from build123d import *

# Parameters (mm, degrees)
SKETCH1_W           = 40
SKETCH1_H           = 40
BOSS_EXTRUDE1_DEPTH = 60
SKETCH2_W           = 20
SKETCH2_H           = 40
CUT_EXTRUDE1_DEPTH  = 30
SKETCH4_W           = 40
SKETCH4_H           = 30
CUT_EXTRUDE2_DEPTH  = 20
SKETCH5_W           = 30
SKETCH5_H           = 10
CUT_EXTRUDE3_DEPTH  = 15
SKETCH6_W           = 15
SKETCH6_H           = 10
CUT_EXTRUDE4_DEPTH  = 25
SKETCH8_W           = 30
SKETCH8_H           = 15
BOSS_EXTRUDE2_DEPTH = 10
SKETCH10_W          = 30
SKETCH10_H          = 25
CUT_EXTRUDE5_DEPTH  = 5
SKETCH11_W          = 30
SKETCH11_H          = 15
CUT_EXTRUDE6_DEPTH  = 5


with BuildPart() as part:
    # Sketch1 → Boss-Extrude1 (new body)
    with BuildSketch(Plane.XY):
        with Locations((20, 20)):
            Rectangle(SKETCH1_W, SKETCH1_H)
    extrude(amount=BOSS_EXTRUDE1_DEPTH)

    # Sketch2 → Cut-Extrude1 (cut)
    with BuildSketch(Plane.XY.offset(60)):
        with Locations((30, 20)):
            Rectangle(SKETCH2_W, SKETCH2_H)
    extrude(amount=-CUT_EXTRUDE1_DEPTH, mode=Mode.SUBTRACT)

    # Sketch4 → Cut-Extrude2 (cut)
    with BuildSketch(Plane(origin=(0, 40, 0), x_dir=(1, 0, 0), z_dir=(0, 1, 0))):
        with Locations((20, -15)):
            Rectangle(SKETCH4_W, SKETCH4_H)
    extrude(amount=-CUT_EXTRUDE2_DEPTH, mode=Mode.SUBTRACT)

    # Sketch5 → Cut-Extrude3 (cut)
    with BuildSketch(Plane(origin=(40, 0, 0), x_dir=(0, 0, -1), z_dir=(1, 0, 0))):
        with Locations((-15, 5)):
            Rectangle(SKETCH5_W, SKETCH5_H)
    extrude(amount=-CUT_EXTRUDE3_DEPTH, mode=Mode.SUBTRACT)

    # Sketch6 → Cut-Extrude4 (cut)
    with BuildSketch(Plane(origin=(20, 0, 0), x_dir=(0, 0, -1), z_dir=(1, 0, 0))):
        with Locations((-52.5, 35)):
            Rectangle(SKETCH6_W, SKETCH6_H)
    extrude(amount=-CUT_EXTRUDE4_DEPTH, mode=Mode.SUBTRACT)

    # Sketch8 → Boss-Extrude2 (add)
    with BuildSketch(Plane(origin=(20, 0, 0), x_dir=(0, 0, -1), z_dir=(1, 0, 0))):
        with Locations((-45, 7.5)):
            Rectangle(SKETCH8_W, SKETCH8_H)
    extrude(amount=BOSS_EXTRUDE2_DEPTH)

    # Sketch10 → Cut-Extrude5 (cut)
    with BuildSketch(Plane(origin=(20, 0, 0), x_dir=(0, 0, -1), z_dir=(1, 0, 0))):
        with Locations((-45, 27.5)):
            Rectangle(SKETCH10_W, SKETCH10_H)
    extrude(amount=-CUT_EXTRUDE5_DEPTH, mode=Mode.SUBTRACT)

    # Sketch11 → Cut-Extrude6 (cut)
    with BuildSketch(Plane(origin=(30, 0, 0), x_dir=(0, 0, -1), z_dir=(1, 0, 0))):
        with Locations((-45, 7.5)):
            Rectangle(SKETCH11_W, SKETCH11_H)
    extrude(amount=-CUT_EXTRUDE6_DEPTH, mode=Mode.SUBTRACT)


solid = part.part
Verification items for the finished model (mm, model axes). A direction names the side the tool comes from. Round coordinates to 2 decimals unless told otherwise and drop trailing zeros. Loops run counter-clockwise (first coordinate to the right, second up) from the corner with the lowest first, then second, coordinate; pieces in that order, holes last. Notation, with made-up numbers: (-4.5, 32) - (46.5, 32) arc R19 ccw to (46.5, 41) - close; hole circle Ø11 at (14, 80). An arc over 180 degrees is marked (long way). Write item = value, one per line.
Q1. Sectioned sample at C-C on y = 16. Record the boundary of the cut face in (x, z), plus the area to 3 significant figures.
Here are the results:
outline = (0, 0) - (40, 0) - (40, 30) - (15, 30) - (15, 60) - (0, 60) - close
area = 1,650 mm^2
Q2. Sectioned sample at A-A on x = 4. Record the boundary of the cut face in (y, z), plus the area to 3 significant figures.
Here are the results:
outline = (0, 0) - (20, 0) - (20, 30) - (40, 30) - (40, 45) - (30, 45) - (30, 60) - (0, 60) - close
area = 1,650 mm^2
Q3. Depth check by flat-ended pin: pin 1 (8 mm diameter, centred on x = 33.5, z = 12, fed in from +Y); pin 2 (4.5 mm diameter, centred on x = 6.5, y = 35, fed in from -Z); pin 3 (5 mm diameter, centred on y = 6.5, z = 38.5, fed in from +X). Enter the tip coordinate at first touch or a pass-through.
Here are the results:
pin_1 = 20
pin_2 = 30
pin_3 = 25
Q4. Tool access check on faces 1 (the flat face through (20, 15, 45)), 2 (the flat face through (8, 35, 45)), 3 (the flat face through (20, 20, 15)), 4 (the flat face through (33, 10, 15)). Record the directions out of +Z, -Z, +X, -X, +Y, -Y that give a thin tool (end or side, any length) a straight path to the whole face; none if there is none.
Here are the results:
face_1 = +Z, +X, +Y
face_2 = +Z, +X, -X, +Y
face_3 = -Z, +X, -X, +Y
face_4 = +Z, -Z, +X, -Y
Q5. Sectioned sample at D-D on y = 22. Record the boundary of the cut face in (x, z).
Here are the results:
outline = (0, 30) - (15, 30) - (15, 60) - (0, 60) - close
Q6. Sectioned sample at B-B on z = 38. Record the boundary of the cut face in (x, y), plus the area to 3 significant figures.
Here are the results:
outline = (0, 0) - (25, 0) - (25, 15) - (15, 15) - (15, 40) - (0, 40) - close
area = 750 mm^2
Q7. Material ranges on L1, parallel to X at y = 8.5, z = 44.5; L2, parallel to X at y = 19, z = 56; L3, parallel to Y at x = 30.5, z = 5, recorded low to high.
Here are the results:
L1 = 0 to 25
L2 = 0 to 15
L3 = 10 to 20
